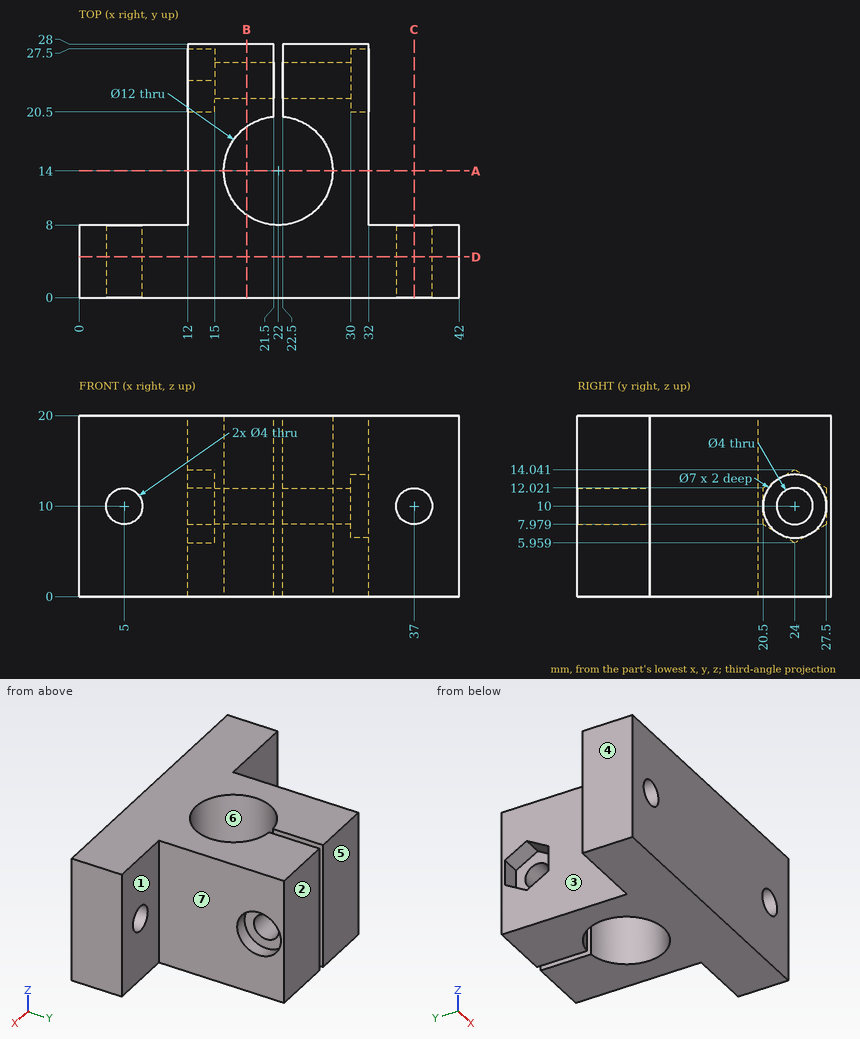
Here's the drawing with two shaded views (mm, measured from the low corner). I have some questions. A direction names the side the tool comes from. Coordinates: 2 decimals unless noted, no trailing zeros. Order: outer loops, then holes, each group sorted by start corner. A loop starts at its lowest first (then second) coordinate and runs counter-clockwise, first axis right, second up.
Item 1: If we section it at D-D, the plane y = 4.5: List the corners of the cut face in (x, z) for me.
Response values:
outline: (0, 0) - (42, 0) - (42, 20) - (0, 20) - close; hole circle Ø4 at (5, 10); hole circle Ø4 at (37, 10)
Item 2: I need wall thicknesses on probe 1 along X at (y, z) = (25.25, 5.25); probe 2 along X at (y, z) = (13.75, 12.5) (1 decimal); probe 3 along Z at (x, y) = (37, 6.25). Which ranges of each line are inside material? Lowest first, please.
Response values:
probe 1: x = 12 to 21.5, 22.5 to 32
probe 2: x = 12 to 16, 28 to 32
probe 3: z = 0 to 8, 12 to 20
Item 3: If we section it at A-A, the plane y = 14: List the corners of the cut face in (x, z) for me.
Response values:
outline: (12, 0) - (16, 0) - (16, 20) - (12, 20) - close; (28, 0) - (32, 0) - (32, 20) - (28, 20) - close
Item 4: Which directions (+Z, -Z, +X, -X, +Y, -Y) give clear straight access to the entire face, cutting with the end or side of a thin tool? Please do the marked faces 1, 2 and 3.
Response values:
face 1: +Z, -Z, +X, +Y
face 2: +Z, -Z, +X, -X, +Y
face 3: +Z, -Z, -X, +Y
Item 5: If we section it at B-B, the plane x = 18.5: List the corners of the cut face in (y, z) for me.
Response values:
outline: (0, 0) - (9.13, 0) - (9.13, 20) - (0, 20) - close; (18.87, 0) - (28, 0) - (28, 20) - (18.87, 20) - close; hole circle Ø4 at (24, 10)
Item 6: I'm going to push flat-ended pins straight in: pin 1 Ø4 at (x, z) = (35, 8) entering from +Y; pin 2 Ø9 at (y, z) = (24, 10) entering from -X; pin 3 Ø12 at (y, z) = (14.5, 2) entering from +X. Where does each tip first touch, or does it pass through?
Response values:
pin 1: stops at y = 8
pin 2: stops at x = 12
pin 3: stops at x = 32
Item 7: If we section it at C-C, the plane x = 37: List the corners of the cut face in (y, z) for me.
Response values:
outline: (0, 0) - (8, 0) - (8, 8) - (0, 8) - close; (0, 12) - (8, 12) - (8, 20) - (0, 20) - close
Item 8: Thinking about a two-plate mould opening in X: for the marked faces 4, 5, 6 and 7, which applies, pulls with the +X half, pulls with the -X half, needs draft (parallel to the pull), parting line crosses it, or undercut?
Response values:
face 4: pulls with the -X half
face 5: needs draft
face 6: undercut
face 7: pulls with the +X half
